Input: dimensioned drawing with shaded views. Units: mm. Origin: part minimum x, y, z. Round coordinates to 2 decimals unless told otherwise and drop trailing zeros. Loops run counter-clockwise (first coordinate to the right, second up) from the corner with the lowest first, then second, coordinate; pieces in that order, holes last.
1) Section C-C, the plane z = 0.65. Return loops of the section in (x, y).
2) Ray query, line 1 along X through (y, z) = (5.75, 2.1); line 2 along Y through (x, z) = (35, 3.95); line 3 along X through (y, z) = (6.75, 3.45). Return the intervals inside material, ascending.
3) Section B-B, the plane x = 36. Return loops of the section in (y, z).
4) First-contact query: pin 1 (2 mm diameter, centred on x = 31.5, z = 3.5, fed in from -Y). Flat tip, straight axial feed; report the tip coordinate or a pass-through.
5) Section A-A, the plane y = 4.5. Return loops of the section in (x, z).
6) Draft query along X for the marked faces 1, 2 and 3. Return one class per face: pulls with the +X half, pulls with the -X half, needs draft (parallel to the pull), parting line crosses it, or undercut.
7) Section D-D, the plane y = 1.25. Return loops of the section in (x, z), and give its area (3 significant figures).
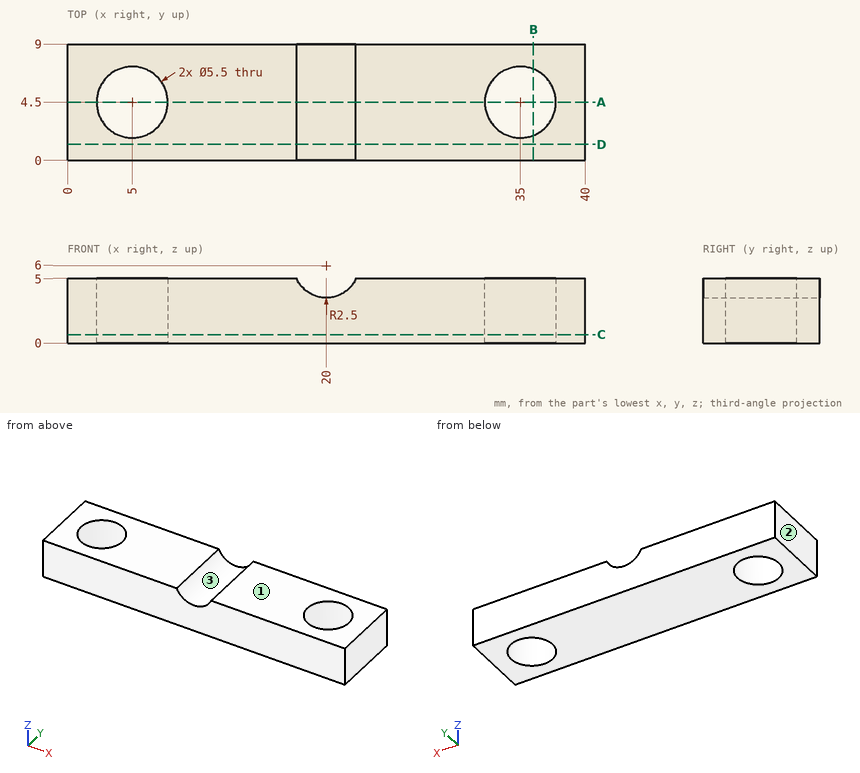
Final values:
1. outline: (0, 0) - (40, 0) - (40, 9) - (0, 9) - close; hole circle Ø5.5 at (5, 4.5); hole circle Ø5.5 at (35, 4.5)
2. line 1: x = 0 to 2.55, 7.45 to 32.55, 37.45 to 40
2. line 2: y = 0 to 1.75, 7.25 to 9
2. line 3: x = 0 to 3.42, 6.58 to 33.42, 36.58 to 40
3. outline: (0, 0) - (1.94, 0) - (1.94, 5) - (0, 5) - close; (7.06, 0) - (9, 0) - (9, 5) - (7.06, 5) - close
4. pin 1: stops at y = 0
5. outline: (0, 0) - (2.25, 0) - (2.25, 5) - (0, 5) - close; (7.75, 0) - (32.25, 0) - (32.25, 5) - (22.29, 5) arc R2.5 cw to (17.71, 5) - (7.75, 5) - close; (37.75, 0) - (40, 0) - (40, 5) - (37.75, 5) - close
6. face 1: needs draft
6. face 2: pulls with the -X half
6. face 3: undercut
7. outline: (0, 0) - (40, 0) - (40, 5) - (22.29, 5) arc R2.5 cw to (17.71, 5) - (0, 5) - close
7. area: 195 mm2
